Can you work these out from the model? Positions are in its coordinate system, mm. A direction names the side the tool comes from. Coordinates: 2 decimals unless noted, no trailing zeros. Order: outer loops, then holes, each group sorted by start corner. A loop starts at its lowest first (then second) coordinate and runs counter-clockwise, first axis right, second up. Notation, with made-up numbers: (72, 75) -> (121, 75) arc R28 ccw to (121, 102) -> close; hole circle Ø8 at (84, 59.25). An arc over 180 degrees is marked (long way). Answer as a JSON object with one key per item and string values. Group by question number.
(1) I need wall thicknesses on line 1 (X direction, y = -3, z = 5.25); line 2 (X direction, y = 7.25, z = 2); line 3 (Z direction, x = -6.45, y = 9). Which ranges of each line are inside material? Lowest first, please.
(2) I want a section at C-C, the plane x = -2.5. List the corners of the cut face in (y, z) for me.
(3) I want a section at D-D, the plane y = 1.25. List the corners of the cut face in (x, z) for me, plus the area to 3 significant figures.
(4) I want a section at A-A, the plane z = 3.5. State how many separate pieces and enclosed holes the cut face has, plus the area to 3 significant figures.
(5) I want a section at B-B, the plane y = -7. List the corners of the cut face in (x, z) for me.
(6) For pin 1 (0.5 mm diameter, centred on x = 4.5, z = 1, fed in from +Y); pin 2 (1.5 mm diameter, centred on x = 1, z = 2.5, fed in from +Y); pin 3 (0.6 mm diameter, centred on x = 6.5, z = 4.5, fed in from -Y), each with a flat end and sliding along its axis, tell me the tip position at first contact or that it passes through.
(7) If we mould it in two halves opening along X, with no side actions, what happens to faces 5 (the flat face through (-7.5, 4, 4)), 6 (the flat face through (0, -2, 1)), 7 (the cylindrical face through (6.49, -10.33, 2.81)), 8 (the flat face through (3.995, 3, 1))? For each: pulls with the +X half, pulls with the -X half, needs draft (parallel to the pull), parting line crosses it, or undercut.
(8) Which directions (+Z, -Z, +X, -X, +Y, -Y) give clear straight access to the entire face, cutting with the end or side of a thin tool? Please do faces 1 (the flat face through (0, 0, 2)), 2 (the flat face through (-5, 4, 6)), 3 (the flat face through (6, -4, 4)), 4 (the flat face through (-0.1, -0.5, 0.5)).
from build123d import *

# Parameters (mm, degrees)
SKETCH_1_W          = 15
SKETCH_1_H          = 25
EXTRUDE_1_DEPTH     = 2
SKETCH_2_W          = 2
SKETCH_2_H          = 25
EXTRUDE_2_DEPTH     = 5
SKETCH_4_W          = 13
SKETCH_4_H          = 4
SKETCH_4_W_2        = 2
EXTRUDE_3_DEPTH     = 2
SKETCH_5_W          = 11
SKETCH_5_H          = 8.5
CUT_EXTRUDE_1_DEPTH = 2
SKETCH_6_W          = 7.990156946
SKETCH_6_H          = 2
CUT_EXTRUDE_2_DEPTH = 17.170961629
CUT_EXTRUDE_3_DEPTH = 21.742468513
FILLET_1_RADIUS     = 3.5
FILLET_1_LENGTH     = 2
FILLET_2_RADIUS     = 3.5
FILLET_2_LENGTH     = 2
SKETCH_9_R          = 1.5
CUT_EXTRUDE_4_DEPTH = 21.742468513
SKETCH_13_W         = 2
SKETCH_13_H         = 8.5
CUT_EXTRUDE_7_DEPTH = 7
SKETCH_14_W         = 1.504921527
SKETCH_14_H         = 2
EXTRUDE_8_DEPTH     = 7
FILLET_3_RADIUS     = 3.5
FILLET_3_LENGTH     = 2
FILLET_4_RADIUS     = 3.5
FILLET_4_LENGTH     = 2
SKETCH_15_R         = 1.5
EXTRUDE_9_DEPTH     = 2
EXTRUDE_START       = 2
SKETCH_16_R         = 1.5
EXTRUDE_10_DEPTH    = 2


with BuildPart() as part:
    # Эскиз1 → Бобышка-Вытянуть1 (new body)
    with BuildSketch(Plane.XY):
        Rectangle(SKETCH_1_W, SKETCH_1_H)
    extrude(amount=EXTRUDE_1_DEPTH)

    # Эскиз2 → Бобышка-Вытянуть2 (add)
    with BuildSketch(Plane.XY.offset(2)):
        with Locations((-6.5, 0)):
            Rectangle(SKETCH_2_W, SKETCH_2_H)
        with Locations((6.5, 0)):
            Rectangle(SKETCH_2_W, SKETCH_2_H)
    extrude(amount=EXTRUDE_2_DEPTH)

    # Эскиз4 → Бобышка-Вытянуть3 (add)
    with BuildSketch(Plane.XY.offset(7)):
        with Locations((-1, 2)):
            Rectangle(SKETCH_4_W, SKETCH_4_H)
        with Locations((-1, -2)):
            Rectangle(SKETCH_4_W, SKETCH_4_H)
        with Locations((6.5, -2)):
            Rectangle(SKETCH_4_W_2, SKETCH_4_H)
        with Locations((6.5, 2)):
            Rectangle(SKETCH_4_W_2, SKETCH_4_H)
    extrude(amount=-EXTRUDE_3_DEPTH)

    # Эскиз5 → Вырез-Вытянуть1 (cut)
    with BuildSketch(Plane(origin=(0, 0, 0), x_dir=(-1, 0, 0), z_dir=(0, 0, -1))):
        with Locations((0, 8.25)):
            Rectangle(SKETCH_5_W, SKETCH_5_H)
        with Locations((0, -8.25)):
            Rectangle(SKETCH_5_W, SKETCH_5_H)
    extrude(amount=-CUT_EXTRUDE_1_DEPTH, mode=Mode.SUBTRACT)

    # Эскиз6 → Вырез-Вытянуть2 (cut, through all)
    with BuildSketch(Plane.XY.offset(7)):
        with Locations((0, 3)):
            Rectangle(SKETCH_6_W, SKETCH_6_H)
        with Locations((0, -3)):
            Rectangle(SKETCH_6_W, SKETCH_6_H)
    extrude(amount=-CUT_EXTRUDE_2_DEPTH, mode=Mode.SUBTRACT)

    # Эскиз8 → Вырез-Вытянуть3 (cut, through all)
    with BuildSketch(Plane.ZY.offset(7.5)):
        Polygon((7, -1), (7, 0), (6, 0), align=None)
        Polygon((6, 0), (7, 0), (7, 1), align=None)
        Polygon((0, -1), (1, 0), (0, 0), align=None)
        Polygon((0, 0), (1, 0), (0, 1), align=None)
    extrude(amount=-CUT_EXTRUDE_3_DEPTH, mode=Mode.SUBTRACT)

    # Скругление1: full round fillet: the end face becomes a half cylinder, R = half its width
    fillet_1_face = Plane((-6.5, 12.5, 3.5), x_dir=(1, 0, 0), z_dir=(0, 1, 0))  # on the end face: x along it, z out of the body
    fillet_1_slab = fillet_1_face.offset(-FILLET_1_RADIUS / 2) * Box(FILLET_1_LENGTH, 2 * FILLET_1_RADIUS, FILLET_1_RADIUS, mode=Mode.PRIVATE)  # the body's end, R deep
    fillet_1_round = Plane((-6.5, 9, 3.5), x_dir=(0, 1, 0), z_dir=(1, 0, 0)) * Cylinder(FILLET_1_RADIUS, FILLET_1_LENGTH, mode=Mode.PRIVATE)  # its axis R under the face
    add(fillet_1_slab - fillet_1_round, mode=Mode.SUBTRACT)

    # Скругление2: full round fillet: the end face becomes a half cylinder, R = half its width
    fillet_2_face = Plane((6.5, 12.5, 3.5), x_dir=(1, 0, 0), z_dir=(0, 1, 0))  # on the end face: x along it, z out of the body
    fillet_2_slab = fillet_2_face.offset(-FILLET_2_RADIUS / 2) * Box(FILLET_2_LENGTH, 2 * FILLET_2_RADIUS, FILLET_2_RADIUS, mode=Mode.PRIVATE)  # the body's end, R deep
    fillet_2_round = Plane((6.5, 9, 3.5), x_dir=(0, 1, 0), z_dir=(1, 0, 0)) * Cylinder(FILLET_2_RADIUS, FILLET_2_LENGTH, mode=Mode.PRIVATE)  # its axis R under the face
    add(fillet_2_slab - fillet_2_round, mode=Mode.SUBTRACT)

    # Эскиз9 → Вырез-Вытянуть4 (cut, through all)
    with BuildSketch(Plane.ZY.offset(7.5)):
        with Locations(Location((3.5, 9, 0), (0, 0, 270))):
            Circle(SKETCH_9_R)
    extrude(amount=-CUT_EXTRUDE_4_DEPTH, mode=Mode.SUBTRACT)

    # Эскиз13 → Вырез-Вытянуть7 (cut)
    with BuildSketch(Plane.XY.offset(7)):
        with Locations((6.5, -8.25)):
            Rectangle(SKETCH_13_W, SKETCH_13_H)
        with Locations((-6.5, -8.25)):
            Rectangle(SKETCH_13_W, SKETCH_13_H)
    extrude(amount=-CUT_EXTRUDE_7_DEPTH, mode=Mode.SUBTRACT)

    # Эскиз14 → Бобышка-Вытянуть8 (add)
    with BuildSketch(Plane.XY.offset(7)):
        Polygon((5.5, -12.5), (5.5, -4), (3.995078473, -4), (3.995078473, -2), (3.5, -2), (3.5, -12.5), align=None)
        with Locations((4.747539236, -3)):
            Rectangle(SKETCH_14_W, SKETCH_14_H)
        Polygon((-3.5, -12.5), (-3.5, -2), (-3.995078473, -2), (-3.995078473, -4), (-5.5, -4), (-5.5, -12.5), align=None)
        with Locations((-4.747539236, -3)):
            Rectangle(SKETCH_14_W, SKETCH_14_H)
    extrude(amount=-EXTRUDE_8_DEPTH)

    # Скругление3: full round fillet: the end face becomes a half cylinder, R = half its width
    fillet_3_face = Plane((-4.5, -12.5, 3.5), x_dir=(1, 0, 0), z_dir=(0, -1, 0))  # on the end face: x along it, z out of the body
    fillet_3_slab = fillet_3_face.offset(-FILLET_3_RADIUS / 2) * Box(FILLET_3_LENGTH, 2 * FILLET_3_RADIUS, FILLET_3_RADIUS, mode=Mode.PRIVATE)  # the body's end, R deep
    fillet_3_round = Plane((-4.5, -9, 3.5), x_dir=(0, -1, 0), z_dir=(1, 0, 0)) * Cylinder(FILLET_3_RADIUS, FILLET_3_LENGTH, mode=Mode.PRIVATE)  # its axis R under the face
    add(fillet_3_slab - fillet_3_round, mode=Mode.SUBTRACT)

    # Скругление4: full round fillet: the end face becomes a half cylinder, R = half its width
    fillet_4_face = Plane((4.5, -12.5, 3.5), x_dir=(-1, 0, 0), z_dir=(0, -1, 0))  # on the end face: x along it, z out of the body
    fillet_4_slab = fillet_4_face.offset(-FILLET_4_RADIUS / 2) * Box(FILLET_4_LENGTH, 2 * FILLET_4_RADIUS, FILLET_4_RADIUS, mode=Mode.PRIVATE)  # the body's end, R deep
    fillet_4_round = Plane((4.5, -9, 3.5), x_dir=(0, -1, 0), z_dir=(-1, 0, 0)) * Cylinder(FILLET_4_RADIUS, FILLET_4_LENGTH, mode=Mode.PRIVATE)  # its axis R under the face
    add(fillet_4_slab - fillet_4_round, mode=Mode.SUBTRACT)

    # Эскиз15 → Бобышка-Вытянуть9 (add)
    with BuildSketch(Plane(origin=(5.5, 0, 0), x_dir=(0, 0, -1), z_dir=(1, 0, 0))):
        with Locations((-3.5, -9)):
            Circle(SKETCH_15_R)
    extrude(amount=EXTRUDE_9_DEPTH)

    # Эскиз16 → Бобышка-Вытянуть10 (add)
    with BuildSketch(Plane.ZY.offset(5.5).offset(EXTRUDE_START)):
        with Locations(Location((3.5, -9, 0), (0, 0, 180))):
            Circle(SKETCH_16_R)
    extrude(amount=-EXTRUDE_10_DEPTH)


solid = part.part
Computed values:
{
 "1": {"line 1": "x = -7.5 to -3.5, 3.5 to 7.5", "line 2": "x = -7.5 to -5.5, 5.5 to 7.5", "line 3": "z = 0 to 2, 5 to 7"},
 "2": {"outline": "(-2, 0) -> (-1, 0) -> (0, 1) -> (1, 0) -> (2, 0) -> (2, 2) -> (-2, 2) -> close; (-2, 5) -> (2, 5) -> (2, 7) -> (1, 7) -> (0, 6) -> (-1, 7) -> (-2, 7) -> close"},
 "3": {"outline": "(-7.5, 0) -> (7.5, 0) -> (7.5, 7) -> (-7.5, 7) -> close; hole (-5.5, 2) -> (5.5, 2) -> (5.5, 5) -> (-5.5, 5) -> close", "area": "72.0 mm2"},
 "4": {"separate pieces": "4", "enclosed holes": "0", "area": "108 mm2"},
 "5": {"outline": "(-5.5, 0) -> (-3.5, 0) -> (-3.5, 7) -> (-5.5, 7) -> close; (3.5, 0) -> (5.5, 0) -> (5.5, 7) -> (3.5, 7) -> close"},
 "6": {"pin 1": "stops at y = 4", "pin 2": "stops at y = 2", "pin 3": "stops at y = -10.33"},
 "7": {"face 5": "pulls with the -X half", "face 6": "undercut", "face 7": "needs draft", "face 8": "undercut"},
 "8": {"face 1": "+Y", "face 2": "+Z, -Z, +Y", "face 3": "+Z, -Z, +X", "face 4": "-Z, +X, -X"}
}
